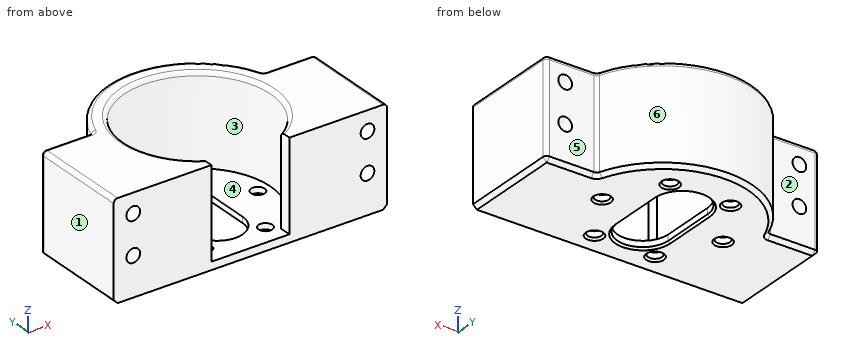
from build123d import *

# Parameters (mm, degrees)
BOX003_W               = 20
BOX003_H               = 4.2
BOX003_DEPTH           = 25
BOX002_W               = 100
BOX002_H               = 4.2
BOX002_DEPTH           = 25
CYLINDER002_R          = 1.75
CYLINDER002_DEPTH      = 60
CYLINDER002_ROLL_ANGLE = -90
ARRAY_X_COUNT          = 2
ARRAY_X_PITCH          = 60
ARRAY_Z_COUNT          = 2
ARRAY_Z_PITCH          = 10
CYLINDER003_R          = 1.75
CYLINDER003_DEPTH      = 10
ARRAY001_COUNT         = 6
CYLINDER005_R          = 6.5
CYLINDER005_DEPTH      = 10
CYLINDER004_R          = 6.5
CYLINDER004_DEPTH      = 10
BOX001_W               = 13
BOX001_H               = 14
BOX001_DEPTH           = 10
CYLINDER001_R          = 18.75
CYLINDER001_DEPTH      = 25
CYLINDER_R             = 23
CYLINDER_DEPTH         = 25
BOX_W                  = 70
BOX_H                  = 30
BOX_DEPTH              = 25
FILLET_R               = 1
CHAMFER_SIZE           = 1
CHAMFER001_SIZE        = 0.5


with BuildPart() as cubo003:
    # Box003 → Box003 (new body)
    with BuildSketch(Plane(origin=(-10, -19, 2), x_dir=(1, 0, 0), z_dir=(0, 0, 1))):
        with Locations((10, 2.1)):
            Rectangle(BOX003_W, BOX003_H)
    extrude(amount=BOX003_DEPTH)


with BuildPart() as fusion003:
    # Box002 → Box002 (new body)
    with BuildSketch(Plane(origin=(-50, -23, 0), x_dir=(1, 0, 0), z_dir=(0, 0, 1))):
        with Locations((50, 2.1)):
            Rectangle(BOX002_W, BOX002_H)
    extrude(amount=BOX002_DEPTH)

    # Fusion003: union Cubo003
    add(cubo003.part)


with BuildPart() as tornillos:
    # Cylinder002 → Cylinder002 (new body)
    with BuildSketch(Plane.XY):
        Circle(CYLINDER002_R)
    extrude(amount=CYLINDER002_DEPTH)


with BuildPart() as tornillos_1:
    # Cylinder002 roll: moved
    add(tornillos.part.rotate(Axis((0, 0, 0), (1, 0, 0)), CYLINDER002_ROLL_ANGLE))


with BuildPart() as tornillos_2:
    # Cylinder002 placement: moved
    add(tornillos_1.part.moved(Location((-30, -30, 10))))

    # Array X: tornillos ×2


with BuildPart() as tornillos_3:
    add(tornillos_2.part)
    with Locations(*[(i * ARRAY_X_PITCH, 0, 0) for i in range(1, ARRAY_X_COUNT)]):
        add(tornillos_2.part)

    # Array Z: tornillos ×2


with BuildPart() as tornillos_4:
    add(tornillos_3.part)
    with Locations(*[(0, 0, i * ARRAY_Z_PITCH) for i in range(1, ARRAY_Z_COUNT)]):
        add(tornillos_3.part)


with BuildPart() as array001:
    # Cylinder003 → Cylinder003 (new body)
    with BuildSketch(Plane(origin=(15.5, 0, 0), x_dir=(1, 0, 0), z_dir=(0, 0, 1))):
        Circle(CYLINDER003_R)
    extrude(amount=CYLINDER003_DEPTH)

    # Array001: Array001 ×6 about axis
    array001_axis = Axis((0, 0, 0), (0, 0, 1))


with BuildPart() as array001_1:
    add(array001.part)
    for i in range(1, ARRAY001_COUNT):
        add(array001.part.rotate(array001_axis, i * 360 / ARRAY001_COUNT))


with BuildPart() as cilindro005:
    # Cylinder005 → Cylinder005 (new body)
    with BuildSketch(Plane(origin=(0, 7, 0), x_dir=(1, 0, 0), z_dir=(0, 0, 1))):
        Circle(CYLINDER005_R)
    extrude(amount=CYLINDER005_DEPTH)


with BuildPart() as cilindro004:
    # Cylinder004 → Cylinder004 (new body)
    with BuildSketch(Plane(origin=(0, -7, 0), x_dir=(1, 0, 0), z_dir=(0, 0, 1))):
        Circle(CYLINDER004_R)
    extrude(amount=CYLINDER004_DEPTH)


with BuildPart() as fusion002:
    # Box001 → Box001 (new body)
    with BuildSketch(Plane(origin=(-6.5, -7, 0), x_dir=(1, 0, 0), z_dir=(0, 0, 1))):
        with Locations((6.5, 7)):
            Rectangle(BOX001_W, BOX001_H)
    extrude(amount=BOX001_DEPTH)

    # Fusion001: union Cilindro005, Cilindro004
    add(cilindro005.part)
    add(cilindro004.part)

    # Fusion002: union Array001
    add(array001_1.part)


with BuildPart() as cilindro001:
    # Cylinder001 → Cylinder001 (new body)
    with BuildSketch(Plane.XY.offset(2)):
        Circle(CYLINDER001_R)
    extrude(amount=CYLINDER001_DEPTH)


with BuildPart() as cilindro:
    # Cylinder → Cylinder (new body)
    with BuildSketch(Plane.XY):
        Circle(CYLINDER_R)
    extrude(amount=CYLINDER_DEPTH)


with BuildPart() as portamotor:
    # Box → Box (new body)
    with BuildSketch(Plane(origin=(-35, -23, 0), x_dir=(1, 0, 0), z_dir=(0, 0, 1))):
        with Locations((35, 15)):
            Rectangle(BOX_W, BOX_H)
    extrude(amount=BOX_DEPTH)

    # Fusion: union Cilindro
    add(cilindro.part)

    # Cut: cut Cilindro001
    add(cilindro001.part, mode=Mode.SUBTRACT)

    # Fillet
    fillet_edges = [portamotor.edges().sort_by_distance(p)[0] for p in [
        (35, -23, 12.5),
        (35, -8, 25),
        (35, 7, 12.5),
        (-35, -23, 12.5),
        (-28.454451, 7, 25),
        (-35, -8, 25),
        (0, 23, 25),
        (28.454451, 7, 25),
        (-18.75, 0, 25),
        (21.908902, 7, 12.5),
        (-35, 7, 12.5),
        (-21.908902, 7, 12.5),
    ]]
    fillet(fillet_edges, radius=FILLET_R)

    # Chamfer
    chamfer_edges = [portamotor.edges().sort_by_distance(p)[0] for p in [
        (35, -8, 0),
        (-28.313708, 7, 0),
        (-34.707107, 6.707107, 0),
        (-22.050067, 7.183503, 0),
        (-35, -8, 0),
        (0, 23, 0),
        (-34.707107, -22.707107, 0),
        (22.050067, 7.183503, 0),
        (0, -23, 0),
        (28.313708, 7, 0),
        (34.707107, -22.707107, 0),
        (34.707107, 6.707107, 0),
    ]]
    chamfer(chamfer_edges, length=CHAMFER_SIZE)

    # Cut001: cut Fusion002
    add(fusion002.part, mode=Mode.SUBTRACT)

    # Cut002: cut tornillos
    add(tornillos_4.part, mode=Mode.SUBTRACT)

    # Chamfer001
    chamfer001_edges = [portamotor.edges().sort_by_distance(p)[0] for p in [
        (13.75, 0, 0),
        (0, 13.5, 0),
        (6.5, 0, 0),
        (0, -13.5, 0),
        (-6.5, 0, 0),
        (-6.875, -11.907849, 0),
        (6.875, 11.907849, 0),
        (-6.875, 11.907849, 0),
        (6.875, -11.907849, 0),
        (-13.75, 0, 0),
    ]]
    chamfer(chamfer001_edges, length=CHAMFER001_SIZE)

    # Cut003: cut Fusion003
    add(fusion003.part, mode=Mode.SUBTRACT)


solid = portamotor.part
Check sheet for the modelled part. Datum: model origin and axes. Units: mm. Face numbers are marked on the shaded views. A direction names the side the tool comes from. Round coordinates to 2 decimals unless told otherwise and drop trailing zeros. Loops run counter-clockwise (first coordinate to the right, second up) from the corner with the lowest first, then second, coordinate; pieces in that order, holes last.
1. Mould release check, pull along X, two halves, no side actions. Record for the marked faces 1, 2 and 3: released by +X, released by -X, zero draft, split by the parting line, or undercut.
2. Sectioned sample at A-A on x = 30. Record the boundary of the cut face in (y, z).
3. Scan lines: probe 1 along Z at (x, y) = (30, -4); probe 2 along X at (y, z) = (-16, 16); probe 3 along X at (y, z) = (-5, 1.5). Record each from-to range of solid material in increasing order.
4. Set-up check for the marked faces 4, 5 and 6: record each of +Z, -Z, +X, -X, +Y, -Y from which the full face is reachable in a straight line by a thin tool's end or side.
5. Sectioned sample at C-C on z = 13.75. Record the boundary of the cut face in (x, y).
6. Sectioned sample at B-B on z = 10. Record the boundary of the cut face in (x, y).
7. Sectioned sample at D-D on y = 5. Give the number of separate pieces and of enclosed holes in the cut face, and give its area (3 significant figures).
8. Gauge pin test, flat ends, axial feed: pin 1 Ø8 at (x, z) = (16.5, 5.5) entering from +Y; pin 2 Ø3.5 at (x, z) = (-28.5, 17.5) entering from +Y; pin 3 Ø1 at (y, z) = (12.5, 21.5) entering from -X. Record the tip position at first contact, or that the pin passes through.
Recorded:
1. face 1: released by -X
1. face 2: zero draft
1. face 3: undercut
2. outline: (-18.8, 0) - (6, 0) - (7, 1) - (7, 8.25) - (-18.8, 8.25) - close; (-18.8, 11.75) - (7, 11.75) - (7, 18.25) - (-18.8, 18.25) - close; (-18.8, 21.75) - (7, 21.75) - (7, 24) arc R1 ccw to (6, 25) - (-18.8, 25) - close
3. probe 1: z = 0 to 8.25, 11.75 to 18.25, 21.75 to 25
3. probe 2: x = -35 to -10, 10 to 35
3. probe 3: x = -35 to -6.5, 6.5 to 35
4. face 4: +Z
4. face 5: +Z, -Z, +X, +Y
4. face 6: +Z, -Z, +Y
5. outline: (-35, -18.8) - (-10, -18.8) - (-10, -15.86) arc R18.75 cw (long way) to (10, -15.86) - (10, -18.8) - (35, -18.8) - (35, 6) arc R1 ccw to (34, 7) - (22.63, 7) arc R1 cw to (21.68, 7.67) arc R23 ccw to (-21.68, 7.67) arc R1 cw to (-22.63, 7) - (-34, 7) arc R1 ccw to (-35, 6) - close
6. outline: (-35, -18.8) - (-31.75, -18.8) - (-31.75, 7) - (-34, 7) arc R1 ccw to (-35, 6) - close; (-28.25, -18.8) - (-10, -18.8) - (-10, -15.86) arc R18.75 cw (long way) to (10, -15.86) - (10, -18.8) - (28.25, -18.8) - (28.25, 7) - (22.63, 7) arc R1 cw to (21.68, 7.67) arc R23 ccw to (-21.68, 7.67) arc R1 cw to (-22.63, 7) - (-28.25, 7) - close; (31.75, -18.8) - (35, -18.8) - (35, 6) arc R1 ccw to (34, 7) - (31.75, 7) - close
7. separate pieces: 2
7. enclosed holes: 4
7. area: 852 mm2
8. pin 1: stops at y = 19.31
8. pin 2: stops at y = 7
8. pin 3: stops at x = -19.62
